For this review, take the finished solid that the model builds, in its own axes (mm). Face numbers are marked on the shaded views. A direction names the side the tool comes from. Round coordinates to 2 decimals unless told otherwise and drop trailing zeros. Write each loop counter-clockwise with the first axis right and the second up, starting at its lowest first coordinate (ties: lowest second). Pieces come first, ordered by that corner, then holes. Notation, with made-up numbers: M 22.25,54.5 L 31.25,54.5 A15 cw 31.25,68.5 Z; hole C -40,-10 d10. An arc over 180 degrees is marked long. One line per question, with ' | ' between items.
Autodesk Inventor part; units mm, degrees
ref_plane "YZ Plane" through (0, 0, 0) normal (1, 0, 0) x (0, 1, 0)
ref_plane "XZ Plane" through (0, 0, 0) normal (0, 1, 0) x (-1, 0, 0)
ref_plane "XY Plane" through (0, 0, 0) normal (0, 0, 1) x (1, 0, 0)
sketch "Sketch1" plane through (0, 0, 0) normal (1, 0, 0) x (0, 1, 0)
  line L0 (0, 0) -> (0, -200)
  line L1 (0, 0) -> (200, 0) construction
  line L2 (0, -200) -> (-240, -200)
  line L3 (-240, -420) -> (0, -420)
  line L4 (0, 0) -> (3, 0)
  line L5 (3, 0) -> (3, -420)
  line L6 (3, -420) -> (-1.1181, -420)
  line L7 (0, -200) -> (0, -420)
  line L8 (-240, -417) -> (0, -417)
  line L9 (-240, -417) -> (0, -417) construction
  line L10 (-240, -200) -> (-265, -200)
  line L11 (-265, -200) -> (-265, -420)
  line L12 (-265, -420) -> (-240, -420)
  line L13 (-240, -417) -> (-265, -417)
  dimension "d0" = 200
  dimension "d1" = 90
  dimension "d2" = 240
  dimension "d3" = 90
  dimension "d4" = 220
  dimension "d8" = 3
  dimension "d9" = 90
  dimension "d10" = 3
  dimension "d18" = 25
  dimension "d19" = 220
  dimension "d20" = 90
extrude "Extrusion4" add sketch "Sketch1" against normal blind 250 contours L4 L5 L6 L7 L0 | L7 L3 L12 L11 L13 L8
extrude "Extrusion5" add sketch "Sketch1" against normal blind 3 contours L7 L8 L13 L11 L10 L2
sketch "Sketch3" plane through (-250, 0, 0) normal (-1, 0, 0) x (0, 0, 1)
  line L0 (-417, -265) -> (-417, 0)
  line L1 (-200, -265) -> (-200, 0)
  line L2 (-417, 0) -> (-200, 0)
  line L3 (-417, -265) -> (-200, -265)
  line L4 (-200, 0) -> (-200, -265)
  line L5 (-200, -265) -> (-417, -265)
  point P0 (0, 0)
extrude "Extrusion6" add sketch "Sketch3" against normal blind 3
properties part number "Pump System Cover"
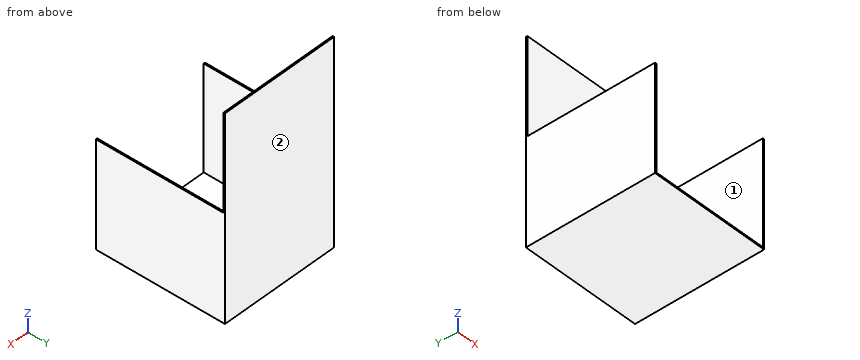
Item 1: To check wall thickness, follow line 1 along X through (y, z) = (-236.5, -267); line 2 along Y through (x, z) = (-125, -180); line 3 along Z through (x, y) = (-43, -220). State the ranges of each line that lie inside material, in increasing order. Write a range as from..to.
Results:
line 1: -250..-247, -3..0 | line 2: 0..3 | line 3: -420..-417
Item 2: Insertion check: pin 1 Ø5 at (x, z) = (-199.5, -365.5) entering from -Y; pin 2 Ø0.9 at (x, y) = (-249, -155.5) entering from +Z. Each pin has a flat end and moves straight along its axis. Give the tip position at first contact, or say it passes through.
Results:
pin 1: y = 0 | pin 2: z = -200
Item 3: Machinability: for the marked faces 1 and 2, which of the approach directions +Z, -Z, +X, -X, +Y, -Y give a long, thin tool a straight path to every point of the face, cutting with its end or side? Answer none if there is none.
Results:
face 1: +Z, -Y | face 2: +Z, -Z, +X, -X, +Y
Item 4: Take a section at D-D (z = -115). Write out the cut boundary in (x, y).
Results:
outline: M -250,0 L 0,0 L 0,3 L -250,3 Z
Item 5: Take a section at C-C (z = -335.5). Write out the cut boundary in (x, y).
Results:
outline: M -250,-265 L -247,-265 L -247,0 L -3,0 L -3,-265 L 0,-265 L 0,3 L -250,3 Z
Item 6: Take a section at B-B (x = -154.5). Write out the cut boundary in (y, z).
Results:
outline: M -265,-420 L 3,-420 L 3,0 L 0,0 L 0,-417 L -265,-417 Z
Item 7: Take a section at A-A (y = -61.5). Write out the cut boundary in (x, z).
Results:
outline: M -250,-420 L 0,-420 L 0,-200 L -3,-200 L -3,-417 L -247,-417 L -247,-200 L -250,-200 Z
